Source: three-view drawing plus pictorial views. Frame: mm from the lowest corner of the part. A direction names the side the tool comes from. Give positions to 0.01 mm unless a question says otherwise; leave off trailing zeros. Order: outer loops, then holes, each group sorted by start corner. A loop starts at its lowest first (then second) coordinate and runs counter-clockwise, first axis right, second up. Notation, with made-up numbers: M 82,9 L 95,9 A15 ccw 95,34 Z; hole C 82,-34 d2. An arc over 180 degrees is marked long. Use CSV: the item, a comma, the result in double quotes. Start each with the question number.
Item 1: Pull-direction query (X, two-part tool) for the marked faces 1 and 2; classes: +X half, -X half, draft (parallel to the pull), parting line (faces both ways), or undercut.
Item 2: Section query B-B on x = 19.5. Return loops of the section in (y, z).
Item 3: First-contact query: pin 1 (2.5 mm diameter, centred on x = 52.5, z = 62.5, fed in from -Y); pin 2 (6 mm diameter, centred on y = 5.5, z = 71.5, fed in from -X); pin 3 (12 mm diameter, centred on x = 11.5, z = 14, fed in from +Y); pin 4 (5 mm diameter, centred on x = 47.5, y = 8.5, fed in from -Z). Flat tips, straight axial feed; report the tip coordinate or a pass-through.
Item 4: Ray query, probe 1 along X at (y, z) = (1.1, 88.5); probe 2 along Z at (x, y) = (52.5, 1.55); probe 3 along Z at (x, y) = (31.5, 7.25). Return the intervals inside material, ascending. Write a range as from..to.
Item 5: Access query for the marked faces 3 and 4. Directions: +Z, -Z, +X, -X, +Y, -Y. A direction counts if a zero-diameter tool reaches every point of the face in a straight line with its end or side. Return the directions, or none.
Item 6: Section query C-C on z = 80.5. Return loops of the section in (x, y).
Item 7: Section query D-D on y = 8.75. Return loops of the section in (x, z), and give its area (3 significant figures).
Item 8: Section query A-A on z = 62.5. Return loops of the section in (x, y).
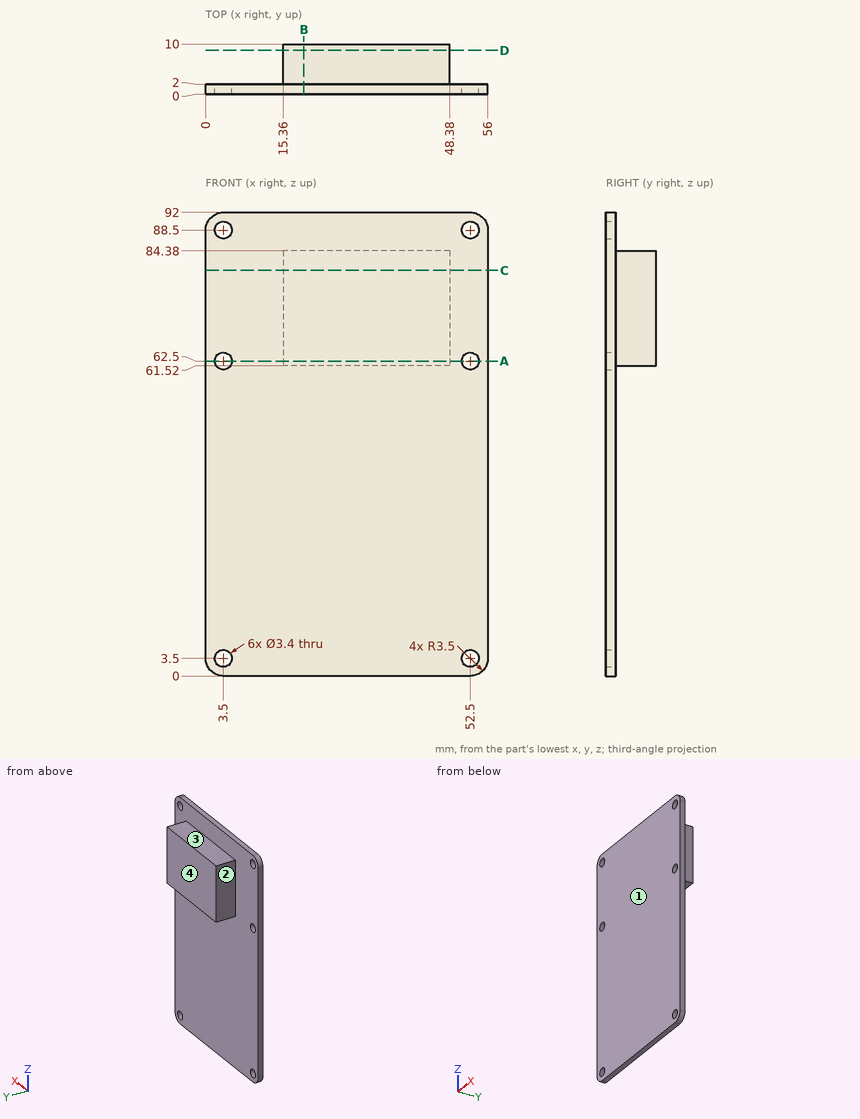
Verdict:
1,face 1,"draft"
1,face 2,"-X half"
2,outline,"M 0,0 L 2,0 L 2,61.52 L 10,61.52 L 10,84.38 L 2,84.38 L 2,92 L 0,92 Z"
3,pin 1,"through"
3,pin 2,"x = 15.36"
3,pin 3,"y = 2"
3,pin 4,"z = 61.52"
4,probe 1,"0..1.8, 5.2..50.8, 54.2..56"
4,probe 2,"0..1.8, 5.2..60.8, 64.2..86.8, 90.2..92"
4,probe 3,"61.52..84.38"
5,face 3,"+Z, +X, -X, +Y"
5,face 4,"+Z, -Z, +X, -X, +Y"
6,outline,"M 0,0 L 56,0 L 56,2 L 48.38,2 L 48.38,10 L 15.36,10 L 15.36,2 L 0,2 Z"
7,outline,"M 15.36,61.52 L 48.38,61.52 L 48.38,84.38 L 15.36,84.38 Z"
7,area,"755 mm2"
8,outline,"M 0,0 L 1.8,0 L 1.8,2 L 0,2 Z; M 5.2,0 L 50.8,0 L 50.8,2 L 48.38,2 L 48.38,10 L 15.36,10 L 15.36,2 L 5.2,2 Z; M 54.2,0 L 56,0 L 56,2 L 54.2,2 Z"
